from build123d import *

# Parameters (mm, degrees)
BOSS_EXTRUDE1_DEPTH      = 14.5
BOSS_EXTRUDE1_DEPTH_BACK = 5.8
BOSS_EXTRUDE2_START      = 13
BOSS_EXTRUDE2_DEPTH      = 1.5
FILLET1_R                = 0.5


with BuildPart() as part:
    # Sketch1 → Boss-Extrude1 (new, two sides: drawn at the far end of the back side and taken through both)
    with BuildSketch(Plane(origin=(72.6, 0, 0), x_dir=(0, 0, -1), z_dir=(1, 0, 0)).offset(-BOSS_EXTRUDE1_DEPTH_BACK)):
        with BuildLine():
            Line((-25.65, 22.55), (-4.35, 22.55))
            ThreePointArc((-4.35, 22.55), (-0.107359313, 20.792640687), (1.65, 16.55))
            Line((1.65, 16.55), (1.65, -2.75))
            ThreePointArc((1.65, -2.75), (-0.107359313, -6.992640687), (-4.35, -8.75))
            Line((-4.35, -8.75), (-25.65, -8.75))
            ThreePointArc((-25.65, -8.75), (-29.892640687, -6.992640687), (-31.65, -2.75))
            Line((-31.65, -2.75), (-31.65, 16.55))
            ThreePointArc((-31.65, 16.55), (-29.892640687, 20.792640687), (-25.65, 22.55))
        make_face()
        with BuildLine():
            Line((-25.6, 19.55), (-4.4, 19.55))
            ThreePointArc((-4.4, 19.55), (-2.950431099, 18.949568901), (-2.35, 17.5))
            Line((-2.35, 17.5), (-2.35, -3.7))
            ThreePointArc((-2.35, -3.7), (-2.950431099, -5.149568901), (-4.4, -5.75))
            Line((-4.4, -5.75), (-25.6, -5.75))
            ThreePointArc((-25.6, -5.75), (-27.049568901, -5.149568901), (-27.65, -3.7))
            Line((-27.65, -3.7), (-27.65, 17.5))
            ThreePointArc((-27.65, 17.5), (-27.049568901, 18.949568901), (-25.6, 19.55))
        make_face(mode=Mode.SUBTRACT)
    extrude(amount=BOSS_EXTRUDE1_DEPTH + BOSS_EXTRUDE1_DEPTH_BACK)

    # Sketch1<4> → Boss-Extrude2 (add)
    with BuildSketch(Plane(origin=(72.6, 0, 0), x_dir=(0, 0, -1), z_dir=(1, 0, 0)).offset(BOSS_EXTRUDE2_START)):
        with BuildLine():
            Line((-4.4, 19.55), (-25.6, 19.55))
            ThreePointArc((-25.6, 19.55), (-27.049568901, 18.949568901), (-27.65, 17.5))
            Line((-27.65, 17.5), (-27.65, -3.7))
            ThreePointArc((-27.65, -3.7), (-27.049568901, -5.149568901), (-25.6, -5.75))
            Line((-25.6, -5.75), (-4.4, -5.75))
            ThreePointArc((-4.4, -5.75), (-2.950431099, -5.149568901), (-2.35, -3.7))
            Line((-2.35, -3.7), (-2.35, 17.5))
            ThreePointArc((-2.35, 17.5), (-2.950431099, 18.949568901), (-4.4, 19.55))
        make_face()
        with BuildLine():
            ThreePointArc((-26.65, 13.55), (-25.185533906, 17.085533906), (-21.65, 18.55))
            Line((-21.65, 18.55), (-8.35, 18.55))
            ThreePointArc((-8.35, 18.55), (-4.814466094, 17.085533906), (-3.35, 13.55))
            Line((-3.35, 13.55), (-3.35, 0.25))
            ThreePointArc((-3.35, 0.25), (-4.814466094, -3.285533906), (-8.35, -4.75))
            Line((-8.35, -4.75), (-21.65, -4.75))
            ThreePointArc((-21.65, -4.75), (-25.185533906, -3.285533906), (-26.65, 0.25))
            Line((-26.65, 0.25), (-26.65, 13.55))
        make_face(mode=Mode.SUBTRACT)
    extrude(amount=BOSS_EXTRUDE2_DEPTH)

    # Fillet1
    fillet1_edges = [part.edges().sort_by_distance(p)[0] for p in [
        (66.8, -6.992640687, 29.892640687),
        (66.8, 6.9, 2.35),
        (66.8, 19.55, 15),
        (66.8, 6.9, -1.65),
        (66.8, 18.949568901, 27.049568901),
        (66.8, 6.9, 27.65),
        (87.1, 6.9, -1.65),
        (87.1, 22.55, 15),
        (66.8, -5.149568901, 27.049568901),
        (87.1, 20.792640687, 29.892640687),
        (87.1, 6.9, 31.65),
        (87.1, -6.992640687, 29.892640687),
        (87.1, -8.75, 15),
        (87.1, -6.992640687, 0.107359313),
        (87.1, 20.792640687, 0.107359313),
        (66.8, -5.75, 15),
        (66.8, -5.149568901, 2.950431099),
        (66.8, 18.949568901, 2.950431099),
        (87.1, 6.9, 26.65),
        (87.1, -4.75, 15),
        (87.1, 17.085533906, 25.185533906),
        (87.1, 18.55, 15),
        (87.1, 17.085533906, 4.814466094),
        (87.1, 6.9, 3.35),
        (87.1, -3.285533906, 4.814466094),
        (87.1, -3.285533906, 25.185533906),
        (66.8, 22.55, 15),
        (66.8, 6.9, 31.65),
        (66.8, 20.792640687, 29.892640687),
        (66.8, 20.792640687, 0.107359313),
        (66.8, -6.992640687, 0.107359313),
        (66.8, -8.75, 15),
    ]]
    fillet(fillet1_edges, radius=FILLET1_R)


solid = part.part
Verification items for the finished model (mm, model axes). A direction names the side the tool comes from. Coordinates: 2 decimals unless noted, no trailing zeros. Write each loop counter-clockwise with the first axis right and the second up, starting at its lowest first coordinate (ties: lowest second). Pieces come first, ordered by that corner, then holes. Notation, with made-up numbers: (76, 83.25) - (106, 83.25) arc R22 ccw to (106, 100.25) - close; hole circle Ø7 at (37, 62). An arc over 180 degrees is marked (long way). Answer as a JSON object with one key per item and string values.
(1) Cross-section at B-B on x = 75.75. Record the cut outline in (y, z).
Report:
{"outline": "(-8.75, 4.35) arc R6 ccw to (-2.75, -1.65) - (16.55, -1.65) arc R6 ccw to (22.55, 4.35) - (22.55, 25.65) arc R6 ccw to (16.55, 31.65) - (-2.75, 31.65) arc R6 ccw to (-8.75, 25.65) - close; hole (-5.75, 4.4) arc R2.05 ccw to (-3.7, 2.35) - (17.5, 2.35) arc R2.05 ccw to (19.55, 4.4) - (19.55, 25.6) arc R2.05 ccw to (17.5, 27.65) - (-3.7, 27.65) arc R2.05 ccw to (-5.75, 25.6) - close"}
(2) Thickness scan on line 1 along Y through (x, z) = (72.5, 10); line 2 along Z through (x, y) = (69.5, 1). Record the ranges inside material, lowest first.
Report:
{"line 1": "-8.75 to -5.75, 19.55 to 22.55", "line 2": "-1.65 to 2.35, 27.65 to 31.65"}
(3) Cross-section at A-A on y = 12.5. Record the cut outline in (x, z), plus the area to 3 significant figures.
Report:
{"outline": "(66.8, -1.15) arc R0.5 ccw to (67.3, -1.65) - (86.6, -1.65) arc R0.5 ccw to (87.1, -1.15) - (87.1, 2.85) arc R0.5 ccw to (86.6, 3.35) - (85.6, 3.35) - (85.6, 2.35) - (67.3, 2.35) arc R0.5 ccw to (66.8, 1.85) - close; (66.8, 28.15) arc R0.5 ccw to (67.3, 27.65) - (85.6, 27.65) - (85.6, 26.65) - (86.6, 26.65) arc R0.5 ccw to (87.1, 27.15) - (87.1, 31.15) arc R0.5 ccw to (86.6, 31.65) - (67.3, 31.65) arc R0.5 ccw to (66.8, 31.15) - close", "area": "165 mm^2"}
(4) Mould release check, pull along Z, two halves, no side actions. Record for faces 4 (the cylindrical face through (76.815, -6.946, 0.061)), 5 (the flat face through (77, 7, 31.65)), 6 (the flat face through (76, 19.55, 15)), 7 (the cylindrical face through (86.09, -3.32, 25.15)): pulls with the +Z half, pulls with the -Z half, needs draft (parallel to the pull), parting line crosses it, or undercut.
Report:
{"face 4": "pulls with the -Z half", "face 5": "pulls with the +Z half", "face 6": "undercut", "face 7": "undercut"}
(5) Tool access check on faces 1 (the cylindrical face through (76.815, 20.746, 29.939)), 2 (the flat face through (76, 7, 2.35)), 3 (the flat face through (86, 18.55, 15)). Record the directions out of +Z, -Z, +X, -X, +Y, -Y that give a thin tool (end or side, any length) a straight path to the whole face; none if there is none.
Report:
{"face 1": "+Z, +X, -X, +Y", "face 2": "-X", "face 3": "+X, -X"}
(6) Gauge pin test, flat ends, axial feed: pin 1 Ø1.5 at (x, z) = (70, 2) entering from +Y; pin 2 Ø7.5 at (y, z) = (12.5, 16) entering from -X; pin 3 Ø1.5 at (x, z) = (80.5, 2) entering from -Y. Record the tip position at first contact, or that the pin passes through.
Report:
{"pin 1": "y = 22.33", "pin 2": "through", "pin 3": "y = -8.53"}
(7) Cross-section at C-C on z = 21. Record the cut outline in (x, y), plus the area to 3 significant figures.
Report:
{"outline": "(66.8, -8.25) arc R0.5 ccw to (67.3, -8.75) - (86.6, -8.75) arc R0.5 ccw to (87.1, -8.25) - (87.1, -5.25) arc R0.5 ccw to (86.6, -4.75) - (85.6, -4.75) - (85.6, -5.75) - (67.3, -5.75) arc R0.5 ccw to (66.8, -6.25) - close; (66.8, 20.05) arc R0.5 ccw to (67.3, 19.55) - (85.6, 19.55) - (85.6, 18.55) - (86.6, 18.55) arc R0.5 ccw to (87.1, 19.05) - (87.1, 22.05) arc R0.5 ccw to (86.6, 22.55) - (67.3, 22.55) arc R0.5 ccw to (66.8, 22.05) - close", "area": "124 mm^2"}
